Here's how the part is built. I have some questions about the finished solid (model axes, mm). A direction names the side the tool comes from. Give positions to 0.01 mm unless a question says otherwise; leave off trailing zeros. Write each loop counter-clockwise with the first axis right and the second up, starting at its lowest first coordinate (ties: lowest second). Pieces come first, ordered by that corner, then holes. Notation, with made-up numbers: (2.5, 22.5) - (33.5, 22.5) arc R20 ccw to (33.5, 35.5) - close; hole circle Ø2 at (-20.5, 53). An arc over 180 degrees is marked (long way). Write each question's results on one line, items separated by ' | '. Start each with the question number.
Item 1: Please list where these lines run through material, in increasing order: line 1 along X through (y, z) = (95.4, -692.15); line 2 along Z through (x, y) = (69.5, 95.75); line 3 along Z through (x, y) = (63.5, 94.45).
Item 2: We'd pull the mould along Y, two halves only. Please class faces 3 (the flat face through (60, 96.52, -93)), 4 (the flat face through (65, 93.345, -93)), 5 (the flat face through (63, 73, -711.2)), 6 (the flat face through (53.975, 84, -93)): +Y half, -Y half, draft (parallel to the pull), parting line (faces both ways), or undercut.
Item 3: Which directions (+Z, -Z, +X, -X, +Y, -Y) give clear straight access to the entire face, cutting with the end or side of a thin tool? Please do faces 1 (the flat face through (76.2, 84, -93)), 2 (the flat face through (65, 74.295, -93)).
Item 4: Suppose I cut it at B-B on z = -6. List the corners of the cut face in (x, y) for me (3 decimals).
Item 5: Suppose I cut it at A-A on y = 84.5. List the corners of the cut face in (x, z) for me (3 decimals).
Item 6: Will this pin go through, and if not, where does the flat tip stop? P1, Ø5.5, axis at x = 65, z = -94, coming from the +Y side.
```python
from build123d import *

# Parameters (mm, degrees)
EXTRUDE_THIN1_START             = 508
SKETCH5_W                       = 25.4
SKETCH5_H                       = 25.4
SKETCH5_W_2                     = 19.05
SKETCH5_H_2                     = 19.05
EXTRUDE_THIN1_DEPTH             = 1219.2
F_5_0MM_DOWEL_HOLE1_D           = 5
F_5_0MM_DOWEL_HOLE1_CSINK_D     = 5.05
F_5_0MM_DOWEL_HOLE1_CSINK_ANGLE = 90


with BuildPart() as part:
    # Sketch5 → Extrude-Thin1 (new body)
    with BuildSketch(Plane.XY.offset(EXTRUDE_THIN1_START)):
        with Locations((63.5, 83.82)):
            Rectangle(SKETCH5_W, SKETCH5_H)
        with Locations((63.5, 83.82)):
            Rectangle(SKETCH5_W_2, SKETCH5_H_2, mode=Mode.SUBTRACT)
    extrude(amount=-EXTRUDE_THIN1_DEPTH)

    # Ø5.0mm Dowel Hole1 (through all)
    with Locations(Plane(origin=(0, 96.52, 0), x_dir=(1, 0, 0), z_dir=(0, 1, 0))):
        with Locations((63.5, 107.95), (63.5, 95.25), (57.15, 692.15), (69.85, 692.15)):
            f_5_0mm_dowel_hole1 = CounterSinkHole(F_5_0MM_DOWEL_HOLE1_D / 2, F_5_0MM_DOWEL_HOLE1_CSINK_D / 2, counter_sink_angle=F_5_0MM_DOWEL_HOLE1_CSINK_ANGLE)

    # Mirror1: Ø5.0mm Dowel Hole1 across plane
    add(f_5_0mm_dowel_hole1.mirror(Plane.XY.offset(-101.6)), mode=Mode.SUBTRACT)


solid = part.part
```
Checked values:
1) line 1: x = 50.8 to 54.65, 59.65 to 67.35, 72.35 to 76.2 | line 2: z = -711.2 to -694.63, -689.67 to 486.47, 491.43 to 508 | line 3: z = -711.2 to -110.45, -105.45 to -97.75, -92.75 to 508
2) face 3: +Y half | face 4: undercut | face 5: draft | face 6: undercut
3) face 1: +Z, -Z, +X, +Y, -Y | face 2: +Z, -Z
4) outline: (50.8, 71.12) - (76.2, 71.12) - (76.2, 96.52) - (50.8, 96.52) - close; hole (53.975, 74.295) - (73.025, 74.295) - (73.025, 93.345) - (53.975, 93.345) - close
5) outline: (50.8, -711.2) - (53.975, -711.2) - (53.975, 508) - (50.8, 508) - close; (73.025, -711.2) - (76.2, -711.2) - (76.2, 508) - (73.025, 508) - close
6) P1: stops at y = 96.52
